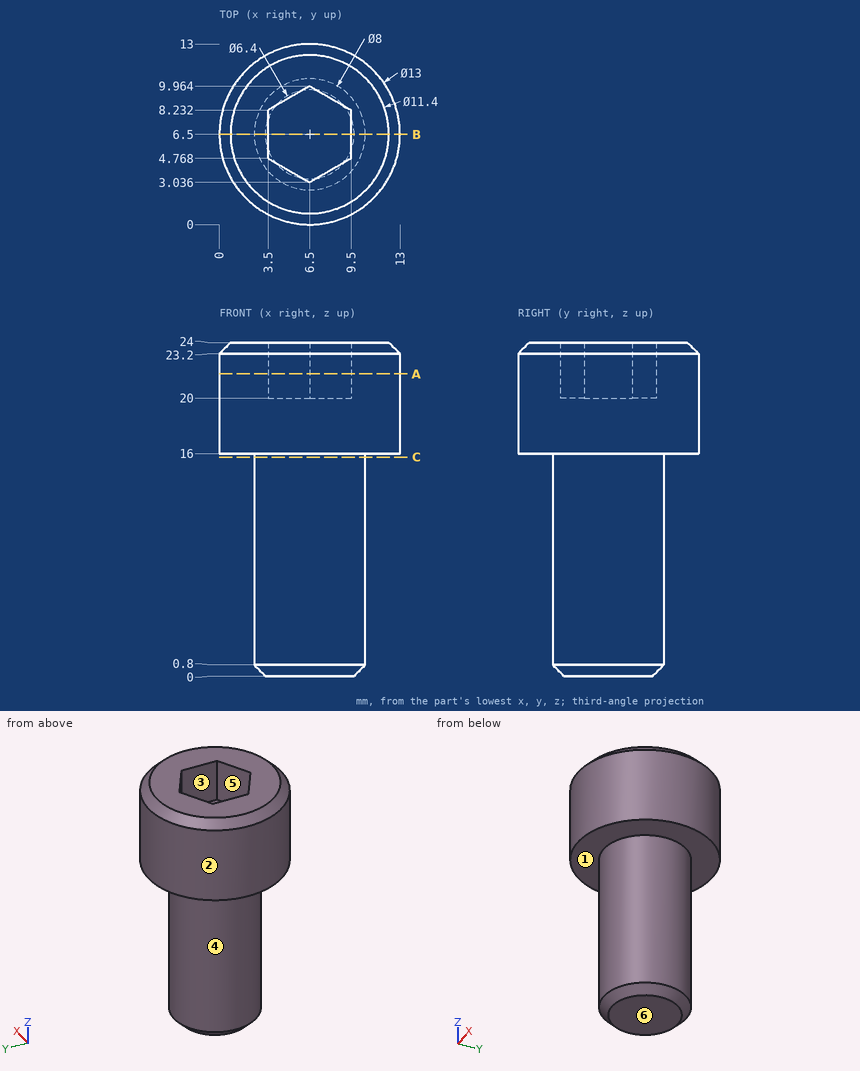
Verification items for this drawing (mm, ordinates from the low corner). A direction names the side the tool comes from. Give positions to 0.01 mm unless a question says otherwise; leave off trailing zeros. Loops run counter-clockwise (first coordinate to the right, second up) from the corner with the lowest first, then second, coordinate; pieces in that order, holes last.
(1) Set-up check for the marked faces 1 and 2: record each of +Z, -Z, +X, -X, +Y, -Y from which the full face is reachable in a straight line by a thin tool's end or side.
From the geometry:
face 1: -Z
face 2: +Z, -Z
(2) Section check C-C on z = 15.75. Record the cut outline in (x, y).
From the geometry:
outline: circle Ø8 at (6.5, 6.5)
(3) Thickness scan on L1, parallel to Z at x = 6.5, y = 7; L2, parallel to Z at x = 2.75, y = 9; L3, parallel to X at y = 3.75, z = 20.5. Record the ranges inside material, lowest first.
From the geometry:
L1: z = 0 to 20
L2: z = 16 to 24
L3: x = 0.61 to 5.26, 7.74 to 12.39
(4) Release check for a two-part mould opening along Y. For the marked faces 3, 4, 5 and 6 record: released by +Y, released by -Y, zero draft, split by the parting line, or undercut.
From the geometry:
face 3: undercut
face 4: split by the parting line
face 5: undercut
face 6: zero draft
(5) Section check B-B on y = 6.5. Record the cut outline in (x, z), then the cut area to 3 significant figures.
From the geometry:
outline: (0, 16) - (2.5, 16) - (2.5, 0.8) - (3.3, 0) - (9.7, 0) - (10.5, 0.8) - (10.5, 16) - (13, 16) - (13, 23.2) - (12.2, 24) - (9.5, 24) - (9.5, 20) - (3.5, 20) - (3.5, 24) - (0.8, 24) - (0, 23.2) - close
area: 207 mm2
(6) Section check A-A on z = 21.75. Record the cut outline in (x, y), then the cut area to 3 significant figures.
From the geometry:
outline: circle Ø13 at (6.5, 6.5); hole (3.5, 4.77) - (6.5, 3.04) - (9.5, 4.77) - (9.5, 8.23) - (6.5, 9.96) - (3.5, 8.23) - close
area: 102 mm2
(7) Depth check by flat-ended pin: pin 1 Ø4 at (x, y) = (8.5, 5.5) entering from -Z; pin 2 Ø2 at (x, z) = (10.5, 4) entering from +Y; pin 3 Ø3 at (y, z) = (10.5, 15.5) entering from +X; pin 4 Ø5 at (x, z) = (5, 3) entering from +Y. Enter the tip coordinate at first touch or a pass-through.
From the geometry:
pin 1: stops at z = 0
pin 2: stops at y = 9.15
pin 3: stops at x = 12.46
pin 4: stops at y = 10.5
